Could you check a few things on this model? Use its own coordinates, in mm. Face numbers are marked on the shaded views. Coordinates: 2 decimals unless noted, no trailing zeros. Loops run counter-clockwise (first coordinate to the right, second up) from the corner with the lowest first, then second, coordinate; pieces in that order, holes last. Notation, with made-up numbers: (-27, 33) -> (28, 33) arc R5 cw to (28, 37) -> close; hole circle Ø7 at (-22.5, -35.5). An arc over 180 degrees is marked (long way). One line per question, with ' | ' between items.
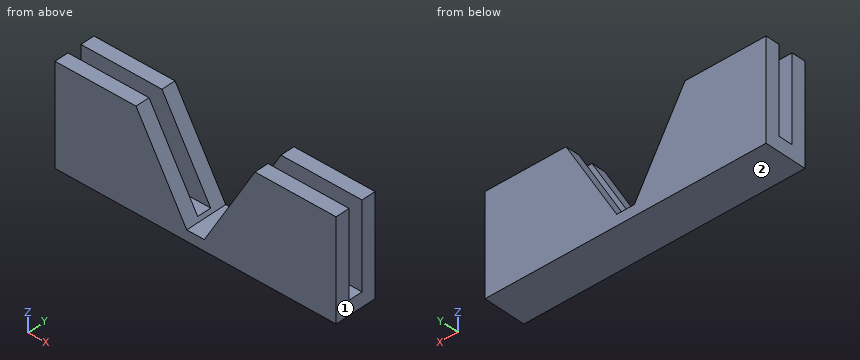
```python
from build123d import *

# Parameters (mm, degrees)
BOSS_EXTRUDE1_DEPTH = 6
SHELL2_START        = 2
SHELL2_OUTLINE_W    = 20
SHELL2_OUTLINE_H    = 2
SHELL2_DEPTH        = 12


# Read off the part's stored shape, not the designer's step: Shell2
with BuildPart() as part:
    # Sketch1 → Boss-Extrude1 (new body)
    with BuildSketch(Plane(origin=(0, 0, 0), x_dir=(1, 0, 0), z_dir=(0, 1, 0))):
        Polygon((0, 0), (0, -14), (11.533121635, -14), (18.75, -1.5), (20, -1.5), (20, 0), align=None)
    extrude(amount=BOSS_EXTRUDE1_DEPTH)

    # Shell2 outline → Shell2 (cut)
    with BuildSketch(Plane.XY.offset(SHELL2_START)):
        with Locations((10, 3)):
            Rectangle(SHELL2_OUTLINE_W, SHELL2_OUTLINE_H)
    extrude(amount=SHELL2_DEPTH, mode=Mode.SUBTRACT)

    # Mirror1: part across plane


with BuildPart() as part_1:
    add(part.part)
    add(part.part.mirror(Plane(origin=(20, 0, 0), x_dir=(0, 0, 1), z_dir=(1, 0, 0))))


solid = part_1.part
```
Q1. Imagine slicing it at D-D on z = 13.25. Write out the boundary of the cut face in (x, y), plus the area to 3 significant figures.
Values follow:
outline: (0, 0) -> (11.97, 0) -> (11.97, 2) -> (0, 2) -> close; (0, 4) -> (11.97, 4) -> (11.97, 6) -> (0, 6) -> close; (28.03, 0) -> (40, 0) -> (40, 2) -> (28.03, 2) -> close; (28.03, 4) -> (40, 4) -> (40, 6) -> (28.03, 6) -> close | area: 95.7 mm2
Q2. Imagine slicing it at B-B on x = 3. Write out the boundary of the cut face in (y, z), plus the area to 3 significant figures.
Values follow:
outline: (0, 0) -> (6, 0) -> (6, 14) -> (4, 14) -> (4, 2) -> (2, 2) -> (2, 14) -> (0, 14) -> close | area: 60.0 mm2
Q3. For pin 1 (6 mm diameter, centred on x = 6.5, z = 4, fed in from -Y); pin 2 (1.2 mm diameter, centred on x = 20.5, y = 3, fed in from +Z), each with a flat end and sliding along its axis, tell me the tip position at first contact or that it passes through.
Values follow:
pin 1: stops at y = 0 | pin 2: stops at z = 1.5
Q4. Please list where these lines run through material, in increasing order: L1, parallel to Y at x = 36, z = 7.25; L2, parallel to X at y = 0.95, z = 2; L3, parallel to Z at x = 21, y = 1.75. Write a range as [from, to].
Values follow:
L1: y = [0, 2], [4, 6] | L2: x = [0, 18.46], [21.54, 40] | L3: z = [0, 1.5]
Q5. Imagine slicing it at C-C on y = 1.35. Write out the boundary of the cut face in (x, z).
Values follow:
outline: (0, 0) -> (40, 0) -> (40, 14) -> (28.47, 14) -> (21.25, 1.5) -> (18.75, 1.5) -> (11.53, 14) -> (0, 14) -> close
Q6. Imagine slicing it at A-A on z = 5.25. Write out the boundary of the cut face in (x, y).
Values follow:
outline: (0, 0) -> (16.58, 0) -> (16.58, 2) -> (0, 2) -> close; (0, 4) -> (16.58, 4) -> (16.58, 6) -> (0, 6) -> close; (23.42, 0) -> (40, 0) -> (40, 2) -> (23.42, 2) -> close; (23.42, 4) -> (40, 4) -> (40, 6) -> (23.42, 6) -> close
Q7. We'd pull the mould along Z, two halves only. Please class the marked faces 1 and 2: released by +Z, released by -Z, zero draft, split by the parting line, or undercut.
Values follow:
face 1: zero draft | face 2: released by -Z
